CAD build for the part. Positions are in the model's coordinates, mm. A direction names the side the tool comes from. Give positions to 0.01 mm unless a question says otherwise; leave off trailing zeros. Write each loop counter-clockwise with the first axis right and the second up, starting at its lowest first coordinate (ties: lowest second). Pieces come first, ordered by that corner, then holes. Notation, with made-up numbers: (35.5, 18.5) - (54.5, 18.5) arc R25 ccw to (54.5, 31.5) - close; hole circle Ø6 at (13, 48). An arc over 180 degrees is marked (long way). Put each result on its own line as item: value. Start each with the question number.
1. Drop flat-ended pins along their axis: pin 1 (2 mm diameter, centred on y = -59, z = -29, fed in from +X); pin 2 (1.5 mm diameter, centred on y = -63.5, z = -9, fed in from -X); pin 3 (6 mm diameter, centred on x = -5.5, y = -25, fed in from +Z). Give the stop position or say it passes through.
2. Tool access for faces 1 (the flat face through (-20.373, -75, -28)), 2 (the flat face through (-3, 0, 0)): list every direction of +Z, -Z, +X, -X, +Y, -Y with a clear straight run to the whole face (end or side of a thin tool).
3. Cut at B-B on x = 6. List the corners of the cut face in (y, z), and give its area (3 significant figures).
4. Cut at C-C on z = 25.5. List the corners of the cut face in (x, y).
5. Cut at A-A on y = -97. List the corners of the cut face in (x, z), and give its area (3 significant figures).
6. Wall check: line 1 (Z direction, x = 28, y = -35.5); line 2 (Z direction, x = 20, y = -88); line 3 (X direction, y = -138, z = -23). Give the ranges that are in metal, low to high.
from build123d import *

# Parameters (mm, degrees)
F1_DEPTH = 152.4


# Not quite as in the source:
# - ends of sketch curves that miss each other by under 0.0002 mm in the source are joined


with BuildPart() as f1:
    # F0 (on Front) → F1 (new body)
    with BuildSketch(Plane.XZ):
        with BuildLine():
            Line((42.688764, 33.7040728), (42.688764, 46.1017112))
            Line((42.688764, 46.1017112), (29.5671748, 46.1017112))
            Line((29.5671748, 46.1017112), (-42.688764, -26.265505))
            Line((-42.688764, -26.265505), (-42.688764, -46.1017112))
            Line((-42.688764, -46.1017112), (-35.2501708, -46.1017112))
            ThreePointArc((-35.2501708, -46.1017112), (-30.8927586674, -35.5819877326), (-20.3730352, -31.2245756))
            Line((-20.3730352, -31.2245756), (-20.3730352, -23.7859824))
            ThreePointArc((-20.3730352, -23.7859824), (0.2093797229, -8.5380689207), (14.0097452821, 13.0416577293))
            ThreePointArc((14.0097452821, 13.0416577293), (25.7531505711, 26.9762086577), (42.688764, 33.7040728))
        make_face()
    extrude(amount=F1_DEPTH)


solid = f1.part
Report:
1. pin 1: stops at x = -20.37
1. pin 2: stops at x = -26.2
1. pin 3: stops at z = 13.99
2. face 1: -Z, +X, +Y, -Y
2. face 2: +Z, -Z, +X, -X, +Y
3. outline: (-152.4, -1.47) - (0, -1.47) - (0, 22.5) - (-152.4, 22.5) - close
3. area: 3,650 mm²
4. outline: (9, -152.4) - (23.84, -152.4) - (23.84, 0) - (9, 0) - close
5. outline: (-42.69, -46.1) - (-35.25, -46.1) arc R14.88 cw to (-20.37, -31.22) - (-20.37, -23.79) arc R70.72 ccw to (14.01, 13.04) arc R37.39 cw to (42.69, 33.7) - (42.69, 46.1) - (29.57, 46.1) - (-42.69, -26.27) - close
5. area: 1,740 mm²
6. line 1: z = 28.47 to 44.53
6. line 2: z = 21.85 to 36.52
6. line 3: x = -39.43 to -18.82
